Geometry check sheet. Reference: the model listing, model coordinates, mm. Face numbers are marked on the shaded views. A direction names the side the tool comes from. Coordinates: 2 decimals unless noted, no trailing zeros. Loops run counter-clockwise (first coordinate to the right, second up) from the corner with the lowest first, then second, coordinate; pieces in that order, holes last. Notation, with made-up numbers: M -4,31 L 11,31 A23 cw 11,58 Z; hole C 5,89 d10. An arc over 180 degrees is marked long. Use CSV: the item, a comma, the result in double quotes.
```python
from build123d import *

# Parameters (mm, degrees)
F2_R     = 2.5
F3_DEPTH = 20


with BuildPart() as f1:
    # F0 (on Front) → F1 (revolve)
    with BuildSketch(Plane.XZ):
        with BuildLine():
            Line((0, -21.435744), (20, -21.435744))
            Line((20, -21.435744), (20, -11.435744))
            Line((20, -11.435744), (14.838474, -11.435744))
            Line((14.838474, -11.435744), (14.838474, -8.435744))
            Line((14.838474, -8.435744), (13, -8.435744))
            Line((13, -8.435744), (13, -6.435744))
            Line((13, -6.435744), (15.020292, -6.435744))
            Line((15.020292, -6.435744), (15.020292, -1.435744))
            Line((15.020292, -1.435744), (13, -1.435744))
            Line((13, -1.435744), (13, 1.564256))
            Line((13, 1.564256), (15, 1.564256))
            Line((15, 1.564256), (15, 8.564256))
            ThreePointArc((15, 8.564256), (7.928932, 11.493188), (5, 18.564256))
            Line((5, 18.564256), (5, 24.564256))
            Line((5, 24.564256), (3.5, 28.564256))
            Line((3.5, 28.564256), (0, 28.564256))
            Line((0, 28.564256), (0, -21.435744))
        make_face()
    revolve(axis=Axis((0, 0, 3.564256), (0, 0, 1)))

    # F2 (on face) → F3 (cut)
    with BuildSketch(Plane.XY.offset(28.564256)):
        Circle(F2_R)
    extrude(amount=-F3_DEPTH, mode=Mode.SUBTRACT)


solid = f1.part
```
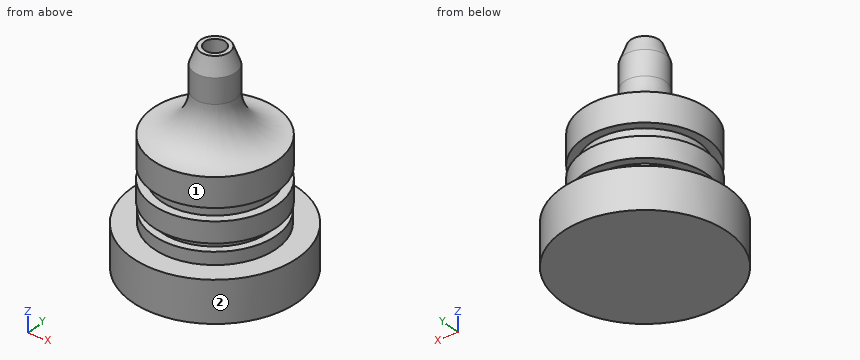
1. Section check D-D, the plane x = -16. Record the cut outline in (y, z).
The answers:
outline,"M -12,-21.44 L 12,-21.44 L 12,-11.44 L -12,-11.44 Z"
2. Section check C-C, the plane z = -16. Record the cut outline in (x, y).
The answers:
outline,"C 0,0 d40"
3. Set-up check for the marked faces 1 and 2: record each of +Z, -Z, +X, -X, +Y, -Y from which the full face is reachable in a straight line by a thin tool's end or side.
The answers:
face 1,"+Z"
face 2,"+Z, -Z"
4. Thickness scan on line 1 (Z direction, x = 14.5, y = 1.5); line 2 (Z direction, x = 13, y = -1); line 3 (Z direction, x = -5.5, y = -15.5). Record the ranges inside material, lowest first. Write a range as [from, to].
The answers:
line 1,"[-21.44, -8.44], [-6.44, -1.44], [1.56, 8.57]"
line 2,"[-21.44, -8.44], [-6.44, -1.44], [1.56, 8.76]"
line 3,"[-21.44, -11.44]"
5. Section check B-B, the plane z = 20.5. Record the cut outline in (x, y).
The answers:
outline,"C 0,0 d10; hole C 0,0 d5"
6. Gauge pin test, flat ends, axial feed: P1, Ø1.5, axis at x = -1, y = 1, coming from the +Z side; P2, Ø1.5, axis at x = -2, y = -13.5, coming from the +Z side; P3, Ø12, axis at x = 13, y = -14, coming from the +Z side. Record the tip position at first contact, or that the pin passes through.
The answers:
P1,"z = 8.56"
P2,"z = 8.79"
P3,"z = 8.75"
